For this review, take the finished solid that the model builds, in its own axes (mm). Face numbers are marked on the shaded views. A direction names the side the tool comes from. Round coordinates to 2 decimals unless told otherwise and drop trailing zeros. Order: outer loops, then holes, each group sorted by start corner. A loop starts at its lowest first (then second) coordinate and runs counter-clockwise, first axis right, second up. Notation, with made-up numbers: (-14.75, 1) - (23.25, 1) arc R23 cw to (23.25, 38) - close; hole circle Ø9 at (77.5, 30.25). An arc over 180 degrees is marked (long way). One line per item, written item: value.
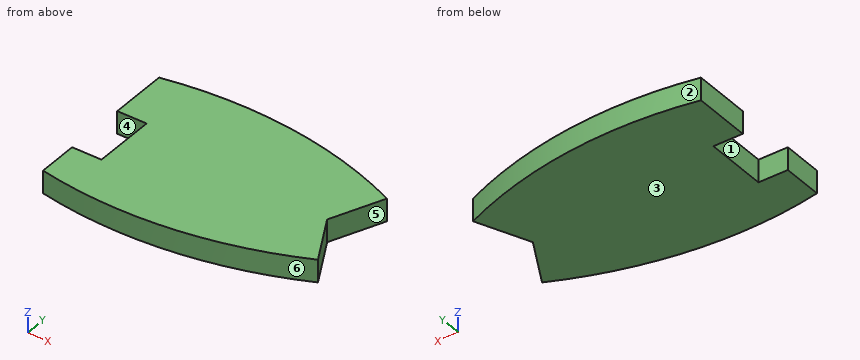
```python
from build123d import *

# Parameters (mm, degrees)
BOSS_EXTRUDE1_DEPTH = 4


with BuildPart() as part:
    # Sketch1 → Boss-Extrude1 (new body)
    with BuildSketch(Plane.XY):
        with BuildLine():
            Line((0, 5.5), (-5.2, 5.5))
            Line((-5.2, 5.5), (-5.2, 15.7))
            ThreePointArc((-5.2, 15.7), (17.140820884, 16.628890564), (38.714781823, 10.751873901))
            Line((38.714781823, 10.751873901), (34.8, 1.55))
            Line((34.8, 1.55), (39.553207037, -7.248126099))
            ThreePointArc((39.553207037, -7.248126099), (17.599991723, -13.46450147), (-5.2, -12.6))
            Line((-5.2, -12.6), (-5.2, -5.5))
            Line((-5.2, -5.5), (0, -5.5))
            Line((0, -5.5), (0, 5.5))
        make_face()
    extrude(amount=BOSS_EXTRUDE1_DEPTH)


solid = part.part
```
Item 1: Take a section at D-D (y = 2.5). Write out the cut boundary in (x, z), plus the area to 3 significant figures.
Returned:
outline: (0, 0) - (35.2, 0) - (35.2, 4) - (0, 4) - close
area: 141 mm^2
Item 2: Take a section at A-A (z = 2.85). Write out the cut boundary in (x, y), plus the area to 3 significant figures.
Returned:
outline: (-5.2, -12.6) arc R73 ccw to (39.55, -7.25) - (34.8, 1.55) - (38.71, 10.75) arc R73 ccw to (-5.2, 15.7) - (-5.2, 5.5) - (0, 5.5) - (0, -5.5) - (-5.2, -5.5) - close
area: 1,140 mm^2
Item 3: The part is to be moulded in two halves that separate along Y. For the marked faces 1, 2 and 3, say which applies: +Y half, -Y half, draft (parallel to the pull), parting line (faces both ways), or undercut.
Returned:
face 1: undercut
face 2: +Y half
face 3: draft
Item 4: For P1, Ø1, axis at x = 27, z = 1, coming from the -Y side; P2, Ø1.2, axis at x = -2, z = 2.5, coming from the +Y side; P3, Ø1, axis at y = -4, z = 1.5, coming from the -X side, all flat-tipped, find the tip position at first contact; note any pin that passes through.
Returned:
P1: y = -11.84
P2: y = 16.35
P3: x = 0
Item 5: Wall thickness on line 1 (Y direction, x = -1, z = 2); line 2 (Y direction, x = 36, z = 1.25); line 3 (X direction, y = 5, z = 3.85): over which ranges is each line inside the solid? List them lowest first.
Returned:
line 1: -13.3 to -5.5, 5.5 to 16.4
line 2: -8.78 to -0.67, 4.37 to 11.9
line 3: 0 to 36.27
Item 6: Take a section at C-C (x = 32). Write out the cut boundary in (y, z).
Returned:
outline: (-10.24, 0) - (13.36, 0) - (13.36, 4) - (-10.24, 4) - close
Item 7: Machinability: for the marked faces 4, 5 and 6, which of the approach directions +Z, -Z, +X, -X, +Y, -Y give a long, thin tool a straight path to every point of the face, cutting with its end or side? Answer none if there is none.
Returned:
face 4: +Z, -Z, -X
face 5: +Z, -Z, +X
face 6: +Z, -Z, -Y
Item 8: Take a section at B-B (x = 37). Write out the cut boundary in (y, z), plus the area to 3 significant figures.
Returned:
outline: (-8.37, 0) - (-2.52, 0) - (-2.52, 4) - (-8.37, 4) - close; (6.72, 0) - (11.49, 0) - (11.49, 4) - (6.72, 4) - close
area: 42.5 mm^2
